Read the model definition and answer for the solid it produces. Units are mm, in the model's axes. Round coordinates to 2 decimals unless told otherwise and drop trailing zeros. Write each loop counter-clockwise with the first axis right and the second up, starting at its lowest first coordinate (ties: lowest second). Pieces come first, ordered by that corner, then holes. Notation, with made-up numbers: (-15.75, 61) - (-7.75, 61) arc R18 cw to (-7.75, 93) - close; hole circle Ø3 at (26, 39.5). An arc over 180 degrees is marked (long way). Use one line per item in the form item = value. Start each with the question number.
1) Consider line 1 along Z through (x, y) = (-25.5, 0.7); line 2 along X through (y, z) = (0.7, -1); line 3 along X through (y, z) = (0.35, -30). Determine where each line is inside the solid, lowest interval first. Write a range as from..to.
2) The part is cut by section D-D, the plane x = 25.5. Give the vertices of the cut face in (y, z).
3) The part is cut by section A-A, the plane z = -36. Give the vertices of the cut face in (x, y), plus the area to 3 significant figures.
4) The part is cut by section B-B, the plane x = 5.5. Give the vertices of the cut face in (y, z), plus the area to 3 significant figures.
5) This flat-tipped pin is pushed along its axis until it touches: pin 1 (4 mm diameter, centred on x = 25.5, z = 44.17, fed in from +Y). Where does it stop, or does it pass through?
6) For a pull along Z with two mould halves and no side action, classify faces 1 (the face through (-46.22, 0.49, -25.94)), 2 (the face through (46.22, 0.49, 25.94)), 3 (the face through (-13, 1, 44)), 4 (the face through (-47.503, 0.507, 0.154)) as released by +Z, released by -Z, zero draft, split by the parting line, or undercut.
7) The part is cut by section C-C, the plane y = 0.35. Give the vertices of the cut face in (x, z).
Autodesk Inventor part; units mm, degrees
ref_plane "YZ Plane" through (0, 0, 0) normal (1, 0, 0) x (0, 1, 0)
ref_plane "XZ Plane" through (0, 0, 0) normal (0, 1, 0) x (-1, 0, 0)
ref_plane "XY Plane" through (0, 0, 0) normal (0, 0, 1) x (1, 0, 0)
sketch "Sketch3" plane through (0, 0, 0) normal (0, 1, 0) x (-1, 0, 0)
  circle A0 centre (0, 0) radius 53
  line L0 (-61.1985, -0.2718) -> (-30.8346, 52.8636)
  line L1 (-30.8346, 52.8636) -> (30.3639, 53.1354)
  line L2 (30.3639, 53.1354) -> (61.1985, 0.2718)
  line L3 (61.1985, 0.2718) -> (30.8346, -52.8636)
  line L4 (30.8346, -52.8636) -> (-30.3639, -53.1354)
  line L5 (-30.3639, -53.1354) -> (-61.1985, -0.2718)
  point P0 (-45.7812, -26.7036)
  dimension "d4" = 106
extrude "Extrusion2" add sketch "Sketch3" along normal blind 1
sketch "Sketch4" plane through (0, 1, 0) normal (0, 1, 0) x (1, 0, 0)
  circle A0 centre (0, 0) radius 45
  dimension "d7" = 90
extrude "Extrusion3" cut sketch "Sketch4" against normal blind 1
sketch "Sketch11" plane through (0, 1, 0) normal (0, 1, 0) x (1, 0, 0)
  line L0 (0, 0) -> (51, 0)
  circle A0 centre (51, 0) radius 3.5
  dimension "d19" = 51
  dimension "d20" = 7
extrude "Extrusion5" cut sketch "Sketch11" against normal blind 10
pattern_circular "Circular Pattern2" count 6 over 360 about axis through (0, 1, 0) along (0, -1, 0) of "Extrusion5"
fillet "Fillet1" radius 2 1 edges at (-30.3639, 0.5, 53.1354)
pattern_circular "Circular Pattern3" count 6 over 360 about axis through (0, 1, 0) along (0, -1, 0) of "Fillet1"
properties part number "crankcase gasket"
Geometry results:
q1.line_1 = -52.89..-47.67, -40.67..-37.08, 37.08..40.67, 47.67..53.11
q1.line_2 = -60.47..-54.35, -47.65..-44.99, 44.99..47.65, 54.35..60.75
q1.line_3 = -43.9..-33.54, 33.54..43.86
q2.outline = (0, -53.11) - (1, -53.11) - (1, -47.67) - (0, -47.67) - close; (0, -40.67) - (1, -40.67) - (1, -37.08) - (0, -37.08) - close; (0, 37.08) - (1, 37.08) - (1, 40.67) - (0, 40.67) - close; (0, 47.67) - (1, 47.67) - (1, 52.89) - (0, 52.89) - close
q3.outline = (-40.47, 0) - (-27, 0) - (-27, 1) - (-40.47, 1) - close; (27, 0) - (40.36, 0) - (40.36, 1) - (27, 1) - close
q3.area = 26.8 mm2
q4.outline = (0, -53.02) - (1, -53.02) - (1, -44.66) - (0, -44.66) - close; (0, 44.66) - (1, 44.66) - (1, 52.98) - (0, 52.98) - close
q4.area = 16.7 mm2
q5.pin_1 = through
q6.face_1 = released by -Z
q6.face_2 = released by +Z
q6.face_3 = zero draft
q6.face_4 = undercut
q7.outline = (-60.63, -0.73) - (-31.41, -51.86) arc R2 ccw to (-29.68, -52.87) - (29.21, -53.13) arc R2 ccw to (30.95, -52.14) - (60.62, -1.27) arc R2 ccw to (60.63, 0.73) - (31.41, 51.86) arc R2 ccw to (29.68, 52.87) - (-29.21, 53.13) arc R2 ccw to (-30.95, 52.14) - (-60.62, 1.27) arc R2 ccw to start; hole circle Ø7 at (-51, 0); hole circle Ø90 at (0, 0); hole circle Ø7 at (-25.5, -44.17); hole circle Ø7 at (-25.5, 44.17); hole circle Ø7 at (25.5, -44.17); hole circle Ø7 at (25.5, 44.17); hole circle Ø7 at (51, 0)
